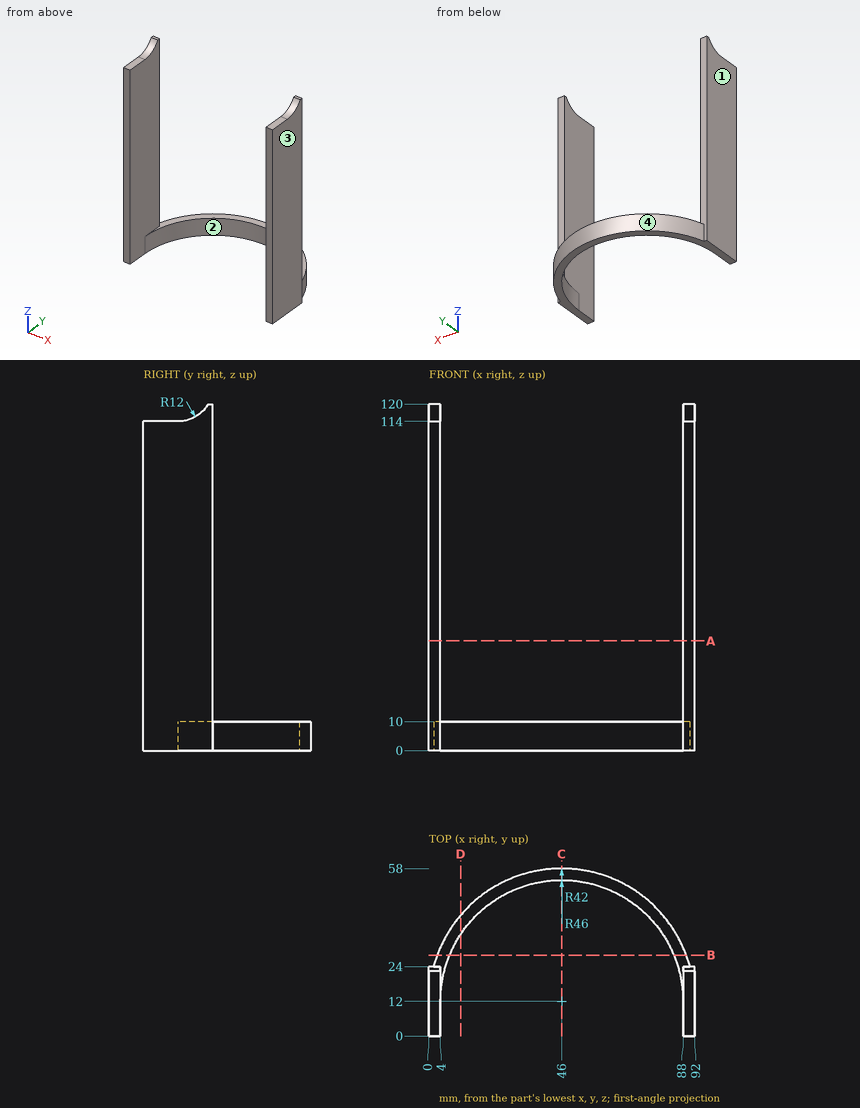
Geometry check sheet. Reference: drawing and pictorial views, mm from the part's lowest x, y, z. Give positions to 0.01 mm unless a question says otherwise; leave off trailing zeros. Loops run counter-clockwise (first coordinate to the right, second up) from the corner with the lowest first, then second, coordinate; pieces in that order, holes last. Notation, with made-up numbers: (28.5, 0) -> (74.5, 0) arc R19 ccw to (74.5, 32) -> close; hole circle Ø8 at (-5, 77.5). An arc over 180 degrees is marked (long way). Answer in a Markdown table with one row per item. Add a question column.
1) Cross-section at D-D on x = 11. Record the boundary of the cut face in (y, z).
2) Material ranges on probe 1 along X at (y, z) = (19, 33); probe 2 along Z at (x, y) = (84.5, 37), recorded low to high. Write a range as from..to.
3) Cross-section at A-A on z = 38. Record the boundary of the cut face in (x, y).
4) Cross-section at B-B on y = 28. Record the boundary of the cut face in (x, z).
5) Draft check along X on the marked faces 1, 2, 3 and 4. Enter one of: pulls with the +X half, pulls with the -X half, needs draft (parallel to the pull), parting line crosses it, or undercut.
6) Gauge pin test, flat ends, axial feed: P1, Ø1.2, axis at x = 2.5, z = 87.5, coming from the +Y side; P2, Ø2, axis at x = 2, y = 9, coming from the +Z side. Record the tip position at first contact, or that the pin passes through.
7) Cross-section at C-C on x = 46. Record the boundary of the cut face in (y, z), and give its area (3 significant figures).
Outcome:
| question | item | result |
|---|---|---|
| 1 | outline | (35.22, 0) -> (41.85, 0) -> (41.85, 10) -> (35.22, 10) -> close |
| 2 | probe 1 | x = 0..4, 88..92 |
| 2 | probe 2 | z = 0..10 |
| 3 | outline | (0, 0) -> (4, 0) -> (4, 24) -> (0, 24) -> close; (88, 0) -> (92, 0) -> (92, 24) -> (88, 24) -> close |
| 4 | outline | (2.87, 0) -> (7.17, 0) -> (7.17, 10) -> (2.87, 10) -> close; (84.83, 0) -> (89.13, 0) -> (89.13, 10) -> (84.83, 10) -> close |
| 5 | face 1 | pulls with the -X half |
| 5 | face 2 | undercut |
| 5 | face 3 | pulls with the +X half |
| 5 | face 4 | parting line crosses it |
| 6 | P1 | stops at y = 24 |
| 6 | P2 | stops at z = 114 |
| 7 | outline | (54, 0) -> (58, 0) -> (58, 10) -> (54, 10) -> close |
| 7 | area | 40.0 mm^2 |
